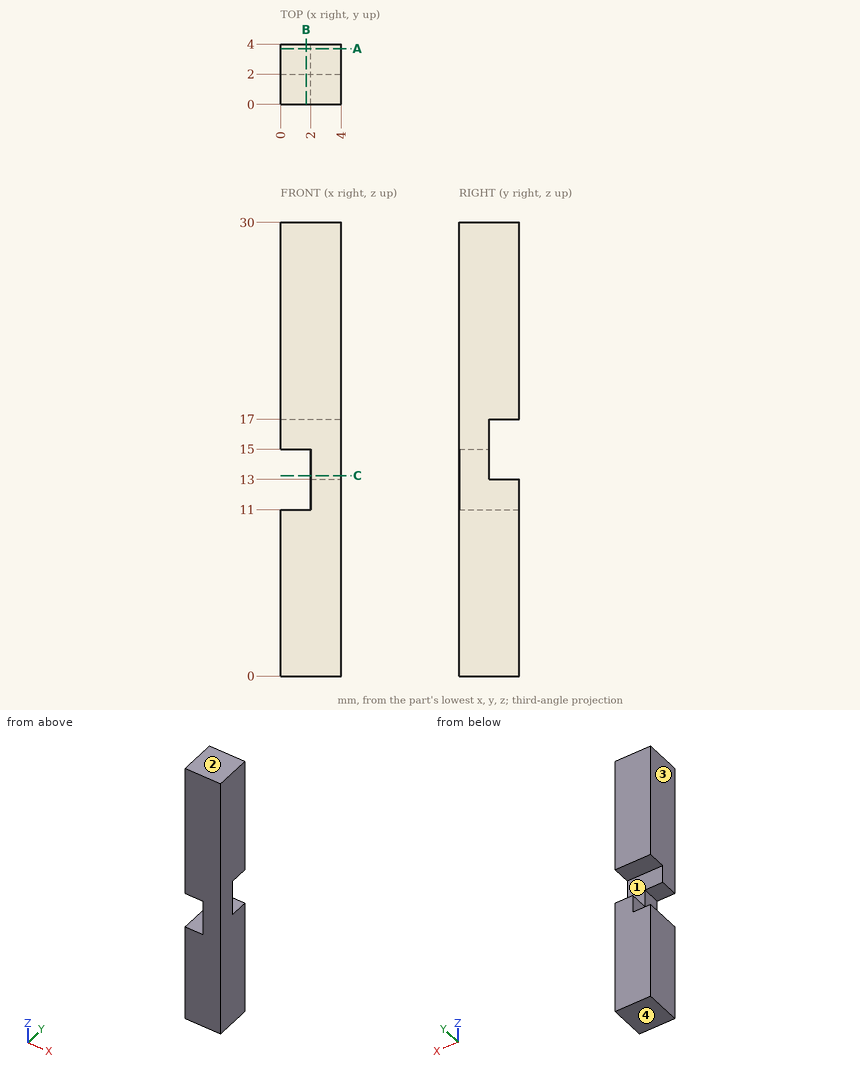
Study the drawing (mm; zero at the part's minimum x, y, z) and answer. Give positions to 0.01 mm unless a question says otherwise; leave off trailing zeros. Order: outer loops, then holes, each group sorted by start corner. A loop starts at its lowest first (then second) coordinate and runs counter-clockwise, first axis right, second up. Notation, with made-up numbers: (83.5, -13) - (106.5, -13) arc R16 cw to (106.5, 2) - close; hole circle Ø4 at (38.25, 22). An arc over 180 degrees is marked (long way). Answer in a Markdown table with one row per item. Add a question column.
Q1. The part is cut by section A-A (y = 3.7). Determine the outline of the cut face in (x, z), then the cut area to 3 significant figures.
Q2. The part is cut by section C-C (z = 13.25). Determine the outline of the cut face in (x, y), then the cut area to 3 significant figures.
Q3. The part is cut by section B-B (x = 1.7). Determine the outline of the cut face in (y, z), then the cut area to 3 significant figures.
Q4. Find the intervals of material crossed by line 1 along Z through (x, y) = (1, 0.4); line 2 along Z through (x, y) = (2.5, 3.75); line 3 along Y through (x, z) = (0.55, 16.75), in increasing order. Write a range as [from, to].
Q5. For a pull along Z with two mould halves and no side action, classify the marked faces 1, 2, 3 and 4 as released by +Z, released by -Z, zero draft, split by the parting line, or undercut.
Determined:
| question | item | result |
|---|---|---|
| 1 | outline | (0, 0) - (4, 0) - (4, 13) - (2, 13) - (2, 11) - (0, 11) - close; (0, 17) - (4, 17) - (4, 30) - (0, 30) - close |
| 1 | area | 100 mm² |
| 2 | outline | (2, 0) - (4, 0) - (4, 2) - (2, 2) - close |
| 2 | area | 4.00 mm² |
| 3 | outline | (0, 0) - (4, 0) - (4, 11) - (0, 11) - close; (0, 15) - (2, 15) - (2, 17) - (4, 17) - (4, 30) - (0, 30) - close |
| 3 | area | 100 mm² |
| 4 | line 1 | z = [0, 11], [15, 30] |
| 4 | line 2 | z = [0, 13], [17, 30] |
| 4 | line 3 | y = [0, 2] |
| 5 | face 1 | undercut |
| 5 | face 2 | released by +Z |
| 5 | face 3 | zero draft |
| 5 | face 4 | released by -Z |
